Verification items for the finished model (mm, model axes). A direction names the side the tool comes from. Give positions to 0.01 mm unless a question says otherwise; leave off trailing zeros. Order: outer loops, then holes, each group sorted by start corner. A loop starts at its lowest first (then second) coordinate and runs counter-clockwise, first axis right, second up.
from build123d import *

# Parameters (mm, degrees)
SKETCH1_W           = 9
SKETCH1_H           = 18
BOSS_EXTRUDE1_DEPTH = 80
SKETCH2_W           = 20
SKETCH2_H           = 15
BOSS_EXTRUDE2_DEPTH = 15
SKETCH4_W           = 9
SKETCH4_H           = 11
CUT_EXTRUDE2_DEPTH  = 20
SKETCH5_R           = 1.6
CUT_EXTRUDE3_DEPTH  = 20
FILLET3_R           = 2
SKETCH6_R           = 1.6
CUT_EXTRUDE4_DEPTH  = 10
CUT_EXTRUDE5_DEPTH  = 10
FILLET8_R           = 1
CHAMFER1_SIZE       = 1.5


with BuildPart() as part:
    # Sketch1 → Boss-Extrude1 (new body)
    with BuildSketch(Plane(origin=(0, 0, 0), x_dir=(1, 0, 0), z_dir=(0, 1, 0))):
        with Locations((-4.5, 9)):
            Rectangle(SKETCH1_W, SKETCH1_H)
    extrude(amount=BOSS_EXTRUDE1_DEPTH)

    # Sketch2 → Boss-Extrude2 (add)
    with BuildSketch(Plane.XZ):
        with Locations((-4.5, -9)):
            Rectangle(SKETCH2_W, SKETCH2_H)
    extrude(amount=BOSS_EXTRUDE2_DEPTH)

    # Sketch4 → Cut-Extrude2 (cut)
    with BuildSketch(Plane(origin=(5.5, 0, 0), x_dir=(0, 0, -1), z_dir=(1, 0, 0))):
        with Locations((9, -9.5)):
            Rectangle(SKETCH4_W, SKETCH4_H)
    extrude(amount=-CUT_EXTRUDE2_DEPTH, mode=Mode.SUBTRACT)

    # Sketch5 → Cut-Extrude3 (cut)
    with BuildSketch(Plane(origin=(0, 0, -16.5), x_dir=(-1, 0, 0), z_dir=(0, 0, -1))):
        with Locations((4.5, -10)):
            Circle(SKETCH5_R)
    extrude(amount=-CUT_EXTRUDE3_DEPTH, mode=Mode.SUBTRACT)

    # Fillet3
    fillet3_edges = [part.edges().sort_by_distance(p)[0] for p in [
        (-9, 80, -9),
        (-4.5, 80, 0),
        (0, 80, -9),
        (-4.5, 80, -18),
    ]]
    fillet(fillet3_edges, radius=FILLET3_R)

    # Sketch6 → Cut-Extrude4 (cut)
    with BuildSketch(Plane(origin=(0, 0, 0), x_dir=(0, 0, -1), z_dir=(1, 0, 0))):
        with Locations((9, 73)):
            Circle(SKETCH6_R)
        with Locations((9, 58)):
            Circle(SKETCH6_R)
        with Locations((9, 43)):
            Circle(SKETCH6_R)
        with Locations((9, 28)):
            Circle(SKETCH6_R)
        with Locations((9, 13)):
            Circle(SKETCH6_R)
    extrude(amount=-CUT_EXTRUDE4_DEPTH, mode=Mode.SUBTRACT)

    # Sketch7 → Cut-Extrude5 (cut)
    with BuildSketch(Plane.ZY.offset(9)):
        Polygon((-16.5, 0), (-18, 3), (-18, 0), align=None)
        Polygon((-1.5, 0), (0, 3), (0, 0), align=None)
    extrude(amount=-CUT_EXTRUDE5_DEPTH, mode=Mode.SUBTRACT)

    # Fillet8
    fillet8_edges = [part.edges().sort_by_distance(p)[0] for p in [
        (0, 0, -9),
        (-9, 0, -9),
    ]]
    fillet(fillet8_edges, radius=FILLET8_R)

    # Chamfer1
    chamfer1_edges = [part.edges().sort_by_distance(p)[0] for p in [
        (-2.9, -10, -1.5),
    ]]
    chamfer(chamfer1_edges, length=CHAMFER1_SIZE)


solid = part.part
(1) Set-up check for faces 1 (the flat face through (-4, -8, -13.5)), 2 (the flat face through (-5, 1, -17)), 3 (the flat face through (-5, -6, -1.5)), 4 (the flat face through (-12, 0, -9)), 5 (the flat face through (0, 39, -9)): record each of +Z, -Z, +X, -X, +Y, -Y from which the full face is reachable in a straight line by a thin tool's end or side.
Solved:
face 1: +X, -X, -Y
face 2: -Z, +X, -X, -Y
face 3: +Z, +X, -X, -Y
face 4: +Z, -Z, -X, +Y
face 5: +Z, -Z, +X, +Y
(2) Scan lines: line 1 (Y direction, x = -4.25, z = -9); line 2 (Y direction, x = -4.5, z = -15.9); line 3 (Y direction, x = -7, z = -8.25). Record each from-to range of solid material in increasing order.
Solved:
line 1: y = -4 to 11.4, 14.6 to 26.4, 29.6 to 41.4, 44.6 to 56.4, 59.6 to 71.4, 74.6 to 80
line 2: y = -15 to -11.6, -8.4 to 80
line 3: y = -4 to 11.59, 14.41 to 26.59, 29.41 to 41.59, 44.41 to 56.59, 59.41 to 71.59, 74.41 to 80
(3) Section check B-B, the plane z = -9. Give the number of separate pieces and of enclosed holes in the cut face, then the cut area to 3 significant figures.
Solved:
separate pieces: 6
enclosed holes: 0
area: 655 mm2
(4) Section check C-C, the plane y = 73. Enter the section's corners in (x, z).
Solved:
outline: (-9, -18) - (0, -18) - (0, -10.6) - (-9, -10.6) - close; (-9, -7.4) - (0, -7.4) - (0, 0) - (-9, 0) - close
(5) Section check A-A, the plane y = -10. Enter the section's corners in (x, z).
Solved:
outline: (-14.5, -16.5) - (-6.1, -16.5) - (-6.1, -13.5) - (-14.5, -13.5) - close; (-14.5, -4.5) - (-6.1, -4.5) - (-6.1, -3) - (-7.6, -1.5) - (-14.5, -1.5) - close; (-2.9, -16.5) - (5.5, -16.5) - (5.5, -13.5) - (-2.9, -13.5) - close; (-2.9, -4.5) - (5.5, -4.5) - (5.5, -1.5) - (-1.4, -1.5) - (-2.9, -3) - close
(6) Go/stop test with flat-tipped pins: pin 1 (9 mm diameter, centred on x = -8, y = -12, fed in from +Z); pin 2 (9 mm diameter, centred on y = 44, z = -7.5, fed in from +X); pin 3 (4 mm diameter, centred on y = 56.5, z = -10, fed in from -X). Record where each tip stops, or that it passes through.
Solved:
pin 1: stops at z = -1.5
pin 2: stops at x = 0
pin 3: stops at x = -9
(7) Release check for a two-part mould opening along Z. For faces 6 (the cylindrical face through (-4.437, 59.586, -8.792)), 7 (the flat face through (-5, 40, 0)), 8 (the cylindrical face through (-4.437, 74.586, -8.792)), 9 (the cylindrical face through (-4.15, -11.56, -15.02)) record: pulls with the +Z half, pulls with the -Z half, needs draft (parallel to the pull), parting line crosses it, or undercut.
Solved:
face 6: undercut
face 7: pulls with the +Z half
face 8: undercut
face 9: needs draft
(8) Section check D-D, the plane x = 3. Enter the section's corners in (y, z).
Solved:
outline: (-15, -16.5) - (0, -16.5) - (0, -1.5) - (-15, -1.5) - (-15, -4.5) - (-4, -4.5) - (-4, -13.5) - (-15, -13.5) - close
